```python
from build123d import *

# Parameters (mm, degrees)
F0_R     = 2.38125
F1_DEPTH = 4.699
F4_D     = 1.778
F4_DEPTH = 8.4790642857
F4_START = 0.3420412
F4_TIP   = 0.5341650903
F7_D     = 1.778
F7_DEPTH = 8.4836
F7_START = 1.0024412
F7_TIP   = 0.5341650903


with BuildPart() as f1:
    # F0 (on Top) → F1 (new body)
    with BuildSketch(Plane.XY):
        with BuildLine():
            Line((9.2692313585, -3.5287562996), (7.6300147115, 2.1878715118))
            ThreePointArc((7.6300147115, 2.1878715118), (-5.6126600757, 5.6126600757), (-2.1878715118, -7.6300147115))
            Line((-2.1878715118, -7.6300147115), (3.5287562996, -9.2692313585))
            ThreePointArc((3.5287562996, -9.2692313585), (5.346264103, -9.3387548259), (6.9889002175, -8.5577844533))
            ThreePointArc((6.9889002175, -8.5577844533), (7.8128228253, -7.8128228253), (8.5577844533, -6.9889002175))
            ThreePointArc((8.5577844533, -6.9889002175), (9.3387548259, -5.346264103), (9.2692313585, -3.5287562996))
        make_face()
        Circle(F0_R, mode=Mode.SUBTRACT)
    extrude(amount=F1_DEPTH)

    # F4
    # its depths count from where the whole tool has entered the part; down to there all is cleared
    with Locations(Plane(origin=(-8.2296, 0, 0), x_dir=(0, 1, 0), z_dir=(-1, 0, 0)).offset(-F4_START)):
        with Locations((0, -2.286)):
            Hole(F4_D / 2, depth=F4_DEPTH)
            with Locations((0, 0, -(F4_DEPTH + F4_TIP / 2))):  # 118° drill point
                Cone(0, F4_D / 2, F4_TIP, mode=Mode.SUBTRACT)

    # F7
    # its depths count from where the whole tool has entered the part; down to there all is cleared
    with Locations(Plane(origin=(0, 8.89, 0), x_dir=(1, 0, 0), z_dir=(0, 1, 0)).offset(-F7_START)):
        with Locations((0, -2.286)):
            Hole(F7_D / 2, depth=F7_DEPTH)
            with Locations((0, 0, -(F7_DEPTH + F7_TIP / 2))):  # 118° drill point
                Cone(0, F7_D / 2, F7_TIP, mode=Mode.SUBTRACT)


solid = f1.part
```
Part model, mm, in its own coordinate system. A direction names the side the tool comes from. Round coordinates to 2 decimals unless told otherwise and drop trailing zeros. Loops run counter-clockwise (first coordinate to the right, second up) from the corner with the lowest first, then second, coordinate; pieces in that order, holes last.
1. Two-plate mould, pull along Z, no slides. Class faces 3 (the face through (1, -3, 4.699)), 4 (the face through (0.116, 5.034, 1.405)), 5 (the face through (9.333, -5.371, 2.317)): pulls with the +Z half, pulls with the -Z half, needs draft (parallel to the pull), parting line crosses it, or undercut.
Solutions:
face 3: pulls with the +Z half
face 4: undercut
face 5: needs draft
2. Slice it at B-B (x = -1.5). Give the cut face in (y, z), and give its area (3 significant figures).
Solutions:
outline: (-7.83, 0) - (-1.85, 0) - (-1.85, 4.7) - (-7.83, 4.7) - close; (1.85, 0) - (7.79, 0) - (7.79, 4.7) - (1.85, 4.7) - close
area: 56.0 mm2
3. Slice it at D-D (z = 1.85). Give the cut face in (x, y) (1 decimal).
Solutions:
outline: (-7.9, -0.8) arc R7.9 ccw to (-2.2, -7.6) - (3.5, -9.3) arc R3.8 ccw to (7, -8.6) arc R11 ccw to (8.6, -7) arc R3.8 ccw to (9.3, -3.5) - (7.6, 2.2) arc R7.9 ccw to (0.8, 7.9) - (0.8, 2.3) arc R2.4 cw (long way) to (-2.3, -0.8) - close; (-7.9, 0.8) - (-2.3, 0.8) arc R2.4 cw to (-0.8, 2.3) - (-0.8, 7.9) arc R7.9 ccw to start
4. Slice it at A-A (z = 3.65). Give the cut face in (x, y) (1 decimal), and give its area (3 significant figures).
Solutions:
outline: (-2.2, -7.6) - (3.5, -9.3) arc R3.8 ccw to (7, -8.6) arc R11 ccw to (8.6, -7) arc R3.8 ccw to (9.3, -3.5) - (7.6, 2.2) arc R7.9 ccw (long way) to start; hole circle Ø4.8 at (0, 0)
area: 209 mm2
5. Slice it at C-C (y = 0). Give the cut face in (x, z) (1 decimal).
Solutions:
outline: (-7.9, 0) - (-2.4, 0) - (-2.4, 1.4) - (-7.9, 1.4) - close; (-7.9, 3.2) - (-2.4, 3.2) - (-2.4, 4.7) - (-7.9, 4.7) - close; (2.4, 0) - (8.3, 0) - (8.3, 4.7) - (2.4, 4.7) - close
6. Drill centre lines: line 1 along Z through (x, y) = (-4.6, 0) (3 decimals); line 2 along X through (y, z) = (5.25, 1.65); line 3 along X through (y, z) = (0.75, 3.4). Where is each one in solid material? Low to high.
Solutions:
line 1: z = 0 to 1.397, 3.175 to 4.699
line 2: x = -5.95 to -0.62, 0.62 to 5.95
line 3: x = -7.9 to -2.26, 2.26 to 8.04
7. 3-axis set-ups, long thin cutter, end or side, ignore diameter. For faces 1 (the face through (1.1, -2.11, 2.32)), 2 (the face through (-5.034, 0.116, 1.405)): which of +Z, -Z, +X, -X, +Y, -Y reach the whole face in a straight line?
Solutions:
face 1: +Z, -Z
face 2: -X
8. Flat gauge pins, fed straight in: pin 1 (1 mm diameter, centred on y = -3.5, z = 4, fed in from -X); pin 2 (1.1 mm diameter, centred on y = 0, z = 2.286, fed in from -X); pin 3 (1.4 mm diameter, centred on x = 0, z = 2.286, fed in from +Y). Where does each tip first touch, or does it go through?
Solutions:
pin 1: stops at x = -7.35
pin 2: stops at x = 2.32
pin 3: stops at y = -2.28
